Autodesk Inventor part; units mm, degrees
ref_plane "YZ Plane" through (0, 0, 0) normal (1, 0, 0) x (0, 1, 0)
ref_plane "XZ Plane" through (0, 0, 0) normal (0, 1, 0) x (-1, 0, 0)
ref_plane "XY Plane" through (0, 0, 0) normal (0, 0, 1) x (1, 0, 0)
sketch "Skizze1" plane through (0, 0, 0) normal (0, 1, 0) x (-1, 0, 0)
  line L0 (12.5, 6) -> (-12.5, 6)
  line L1 (-12.5, 6) -> (-12.5, -6)
  line L2 (-12.5, -6) -> (12.5, -6)
  line L3 (12.5, -6) -> (12.5, 6)
  line L4 (12.5, 6) -> (-12.5, -6) construction
  line L5 (-12.5, 6) -> (12.5, -6) construction
  point P0 (0, 0)
  dimension "d0" = 12
  dimension "d2" = 25
extrude "Extrusion1" add sketch "Skizze1" along normal blind 8
fillet "Rundung1" radius 2 2 edges at (12.5, 4, 6) (12.5, 4, -6)
shell "Wandung1" thickness 1.25 removed faces 2 at (-12.5, 2.6667, -2) at (2.8333, 8, -2)
properties part number "P_Case"
For this review, take the finished solid that the model builds, in its own axes (mm). A direction names the side the tool comes from. Give positions to 0.01 mm unless a question says otherwise; leave off trailing zeros. Order: outer loops, then holes, each group sorted by start corner. A loop starts at its lowest first (then second) coordinate and runs counter-clockwise, first axis right, second up.
1) Wall thickness on line 1 (Z direction, x = -6, y = 5.5); line 2 (Y direction, x = -9.25, z = -2.5); line 3 (X direction, y = 7, z = -4): over which ranges is each line inside the solid? List them lowest first.
2) For faces 1 (the face through (12.5, 4, 0)), 2 (the face through (-1, 5, 4.75)), list the 3-axis set-ups (+Z, -Z, +X, -X, +Y, -Y) from which the entire face can be reached by the end or side of a thin tool; tool diameter is ignored.
3) Insertion check: pin 1 (1.5 mm diameter, centred on y = 6.5, z = -2.5, fed in from -X); pin 2 (5 mm diameter, centred on x = 3.5, z = 2, fed in from +Y). Each pin has a flat end and moves straight along its axis. Give the tip position at first contact, or say it passes through.
4) Take a section at C-C (z = 0.5). Give the boundary of the cut face in (x, y), then the cut area to 3 significant figures.
5) Take a section at B-B (x = -7.25). Give the boundary of the cut face in (y, z).
6) Take a section at A-A (y = 4). Give the boundary of the cut face in (x, z), then the cut area to 3 significant figures.
7) The part is to be moulded in two halves that separate along Z. For faces 3 (the face through (-12.5, 1, 0)), 4 (the face through (-1, 4, -6)), 5 (the face through (0, 1.25, 0)), 6 (the face through (11.9, 4.06, 5.43)), say which applies: released by +Z, released by -Z, zero draft, split by the parting line, or undercut.
Derived:
1. line 1: z = -6 to -4.75, 4.75 to 6
1. line 2: y = 0 to 1.25
1. line 3: x = 11.25 to 12.5
2. face 1: +Z, -Z, +X, +Y, -Y
2. face 2: -X, +Y
3. pin 1: stops at x = 11.25
3. pin 2: stops at y = 1.25
4. outline: (-12.5, 0) - (12.5, 0) - (12.5, 8) - (11.25, 8) - (11.25, 1.25) - (-12.5, 1.25) - close
4. area: 39.7 mm2
5. outline: (0, -6) - (8, -6) - (8, -4.75) - (1.25, -4.75) - (1.25, 4.75) - (8, 4.75) - (8, 6) - (0, 6) - close
6. outline: (-12.5, -6) - (10.5, -6) arc R2 ccw to (12.5, -4) - (12.5, 4) arc R2 ccw to (10.5, 6) - (-12.5, 6) - (-12.5, 4.75) - (10.5, 4.75) arc R0.75 cw to (11.25, 4) - (11.25, -4) arc R0.75 cw to (10.5, -4.75) - (-12.5, -4.75) - close
6. area: 72.9 mm2
7. face 3: zero draft
7. face 4: released by -Z
7. face 5: undercut
7. face 6: released by +Z
